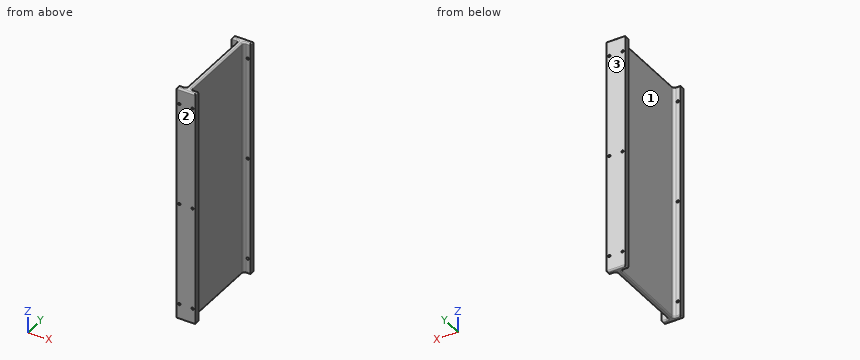
```python
from build123d import *

# Parameters (mm, degrees)
BOSS_EXTRUDE1_DEPTH   = 250
FILLET1_R             = 3
F_5_0MM_DOWEL_HOLE1_D = 5


with BuildPart() as part:
    # Sketch2 → Boss-Extrude1 (new, symmetric)
    with BuildSketch(Plane.XY):
        with BuildLine():
            Line((5, 85), (5, -85))
            ThreePointArc((5, -85), (6.464466094, -88.535533906), (10, -90))
            Line((10, -90), (20, -90))
            Line((20, -90), (20, -100))
            Line((20, -100), (-20, -100))
            Line((-20, -100), (-20, -90))
            Line((-20, -90), (-10, -90))
            ThreePointArc((-10, -90), (-6.464466094, -88.535533906), (-5, -85))
            Line((-5, -85), (-5, 85))
            ThreePointArc((-5, 85), (-6.464466094, 88.535533906), (-10, 90))
            Line((-10, 90), (-20, 90))
            Line((-20, 90), (-20, 100))
            Line((-20, 100), (20, 100))
            Line((20, 100), (20, 90))
            Line((20, 90), (10, 90))
            ThreePointArc((10, 90), (6.464466094, 88.535533906), (5, 85))
        make_face()
    extrude(amount=BOSS_EXTRUDE1_DEPTH, both=True)

    # Fillet1
    fillet1_edges = [part.edges().sort_by_distance(p)[0] for p in [
        (-5, 0, 250),
        (-6.464466094, -88.535533906, 250),
        (-15, 90, -250),
        (-20, 95, -250),
        (0, 100, -250),
        (20, 95, -250),
        (15, 90, -250),
        (6.464466094, 88.535533906, -250),
        (-15, -90, 250),
        (5, 0, -250),
        (6.464466094, -88.535533906, -250),
        (15, -90, -250),
        (20, -95, -250),
        (0, -100, -250),
        (-20, -95, -250),
        (-15, -90, -250),
        (-6.464466094, -88.535533906, -250),
        (-5, 0, -250),
        (-6.464466094, 88.535533906, -250),
        (-20, -95, 250),
        (0, -100, 250),
        (20, -95, 250),
        (15, -90, 250),
        (6.464466094, -88.535533906, 250),
        (5, 0, 250),
        (6.464466094, 88.535533906, 250),
        (-6.464466094, 88.535533906, 250),
        (15, 90, 250),
        (20, 95, 250),
        (0, 100, 250),
        (-20, 95, 250),
        (-15, 90, 250),
    ]]
    fillet(fillet1_edges, radius=FILLET1_R)

    # Ø5.0mm Dowel Hole1 (through all)
    with Locations(Plane(origin=(0, 100, 0), x_dir=(1, 0, 0), z_dir=(0, 1, 0))):
        with Locations((14, 217), (-14, 217), (-14, -217), (14, -217), (-14, 0), (14, 0)):
            Hole(F_5_0MM_DOWEL_HOLE1_D / 2)


solid = part.part
```
The model under review builds one solid part; all positions refer to its coordinate system, in mm. Face numbers are marked on the shaded views. Coordinates: 2 decimals unless noted, no trailing zeros. Order: outer loops, then holes, each group sorted by start corner. A loop starts at its lowest first (then second) coordinate and runs counter-clockwise, first axis right, second up. Notation, with made-up numbers: (53, 20.5) -> (96, 20.5) arc R5 ccw to (96, 28.5) -> close; hole circle Ø6 at (-39, 58). An arc over 180 degrees is marked (long way). Answer in a Markdown table with one row per item. Add a question column.
Item 1: Mouldability with a two-part tool opening along Y and no side actions: class the marked faces 1, 2 and 3 as +Y half, -Y half, draft (parallel to the pull), parting line (faces both ways), or undercut.
Item 2: We need section B-B on z = -13.5. Write out the cut boundary in (x, y), plus the area to 3 significant figures.
Item 3: Clearance check with flat-ended pins moving along their axes: pin 1 (6 mm diameter, centred on y = -63.5, z = 160, fed in from -X); pin 2 (5 mm diameter, centred on y = 0, z = -10.5, fed in from +X). State where each tip first meets the part, or that it passes through.
Item 4: To check wall thickness, follow probe 1 along Z at (x, y) = (-14, 95); probe 2 along X at (y, z) = (-96, 217); probe 3 along Y at (x, z) = (-14.5, -62.5). State the ranges of each line that lie inside material, in increasing order.
Item 5: We need section A-A on y = -80. Write out the cut boundary in (x, z).
Final values:
| question | item | result |
|---|---|---|
| 1 | face 1 | undercut |
| 1 | face 2 | -Y half |
| 1 | face 3 | +Y half |
| 2 | outline | (-20, -100) -> (20, -100) -> (20, -90) -> (10, -90) arc R5 cw to (5, -85) -> (5, 85) arc R5 cw to (10, 90) -> (20, 90) -> (20, 100) -> (-20, 100) -> (-20, 90) -> (-10, 90) arc R5 cw to (-5, 85) -> (-5, -85) arc R5 cw to (-10, -90) -> (-20, -90) -> close |
| 2 | area | 2,620 mm2 |
| 3 | pin 1 | stops at x = -5 |
| 3 | pin 2 | stops at x = 5 |
| 4 | probe 1 | z = -250 to -219.5, -214.5 to -2.5, 2.5 to 214.5, 219.5 to 250 |
| 4 | probe 2 | x = -20 to -16.5, -11.5 to 11.5, 16.5 to 20 |
| 4 | probe 3 | y = -100 to -90, 90 to 100 |
| 5 | outline | (-5, -247) arc R3 ccw to (-2, -250) -> (2, -250) arc R3 ccw to (5, -247) -> (5, 247) arc R3 ccw to (2, 250) -> (-2, 250) arc R3 ccw to (-5, 247) -> close |
